Model file for the job. Use its own axes, mm. Coordinates: 2 decimals unless noted, no trailing zeros. Order: outer loops, then holes, each group sorted by start corner. A loop starts at its lowest first (then second) coordinate and runs counter-clockwise, first axis right, second up. Notation, with made-up numbers: (-19.5, 70) -> (36.5, 70) arc R8 cw to (36.5, 81) -> close; hole circle Ø5 at (-1.75, 18). An arc over 180 degrees is marked (long way). Use CSV: the item, a comma, the result in double quotes. Start each with the question number.
(1) Probe L1, parallel to Y at x = 40.9, z = -0.35; L2, parallel to X at y = 25.5, z = -0.75; L3, parallel to Z at x = -53, y = 20. List the from-to ranges inside material, lowest first.
(2) Cut at B-B on x = -21. Write the cut outline in (y, z), plus the area to 3 significant figures.
(3) Pull direction Y, two halves, no side cores. Call faces 1 (the cylindrical face through (-88.515, 24.98, -0.493)), 2 (the flat face through (-26.05, -0.584, -11.181)), 3 (the flat face through (-26, 18, -1)): pulls with the +Y half, pulls with the -Y half, needs draft (parallel to the pull), parting line crosses it, or undercut.
(4) Cut at C-C on y = -2.5. Write the cut outline in (x, z), plus the area to 3 significant figures.
(5) Pin check, flat tips, straight feed: pin 1 Ø4 at (x, y) = (-90.9, 24.23) entering from +Z; pin 2 Ø12 at (y, z) = (-2, -11) entering from -X; pin 3 Ø11 at (x, y) = (-32, 22.5) entering from -Z; pin 4 Ø6 at (x, y) = (-31.5, 8) entering from -Z. Stop position of each tip, or through.
(6) Cut at A-A on x = 40.9. Write the cut outline in (y, z).
```python
from build123d import *

# Parameters (mm, degrees)
SKETCH1_W            = 150
SKETCH1_H            = 23.35790613
BASE_FLANGE1_DEPTH   = 1
EDGE_FLANGE2_START   = -100
EDGE_FLANGE2_DEPTH   = 150
EDGE_FLANGE2_2_DEPTH = 150
SKETCH13_R           = 2.5
CUT_EXTRUDE1_DEPTH   = 3


# Read off the part's stored shape, not the designer's step: Edge-Flange2
# Sheet-metal steps are written as plain solids
with BuildPart() as part:
    # Sketch1 → Base-Flange1 (new body)
    with BuildSketch(Plane.XY):
        with Locations((-25, 17.550273337)):
            Rectangle(SKETCH1_W, SKETCH1_H)
    extrude(amount=-BASE_FLANGE1_DEPTH)

    # Edge-Flange2 outline → Edge-Flange2 (cut)
    with BuildSketch(Plane.YZ.offset(EDGE_FLANGE2_START)):
        with BuildLine():
            Line((5.871320272, 0), (5.871320272, -0.367006837))
            ThreePointArc((5.871320272, -0.367006837), (6.420209917, -0.093958772), (7.02602081, 0))
            Line((7.02602081, 0), (5.871320272, 0))
        make_face()
    extrude(amount=EDGE_FLANGE2_DEPTH, mode=Mode.SUBTRACT)

    # Edge-Flange2 2 outline → Edge-Flange2 2 (add)
    with BuildSketch(Plane.YZ.offset(EDGE_FLANGE2_START)):
        with BuildLine():
            ThreePointArc((5.871320272, -0.367006837), (5.548352573, -0.652225322), (5.293970003, -1))
            Line((5.293970003, -1), (-6.628679728, -21.650635095))
            Line((-6.628679728, -21.650635095), (-5.762654324, -22.150635095))
            Line((-5.762654324, -22.150635095), (6.159995406, -1.5))
            ThreePointArc((6.159995406, -1.5), (6.52602081, -1.133974596), (7.02602081, -1))
            Line((7.02602081, -1), (5.871320272, -1))
            Line((5.871320272, -1), (5.871320272, -0.367006837))
        make_face()
    extrude(amount=EDGE_FLANGE2_2_DEPTH)

    # Sketch13 → Cut-Extrude1 (cut)
    with BuildSketch(Plane.XY):
        with Locations((40.9, 24.229226402)):
            Circle(SKETCH13_R)
        with Locations((-90.9, 24.229226402)):
            Circle(SKETCH13_R)
    extrude(amount=-CUT_EXTRUDE1_DEPTH, mode=Mode.SUBTRACT)


solid = part.part
```
Outcome:
1,L1,"5.9 to 21.73, 26.73 to 29.23"
1,L2,"-100 to -93.05, -88.75 to 38.75, 43.05 to 50"
1,L3,"-1 to 0"
2,outline,"(-6.63, -21.65) -> (-5.76, -22.15) -> (6.16, -1.5) arc R1 cw to (7.03, -1) -> (29.23, -1) -> (29.23, 0) -> (7.03, 0) arc R2 ccw to (5.29, -1) -> close"
2,area,"47.6 mm2"
3,face 1,"undercut"
3,face 2,"pulls with the -Y half"
3,face 3,"needs draft"
4,outline,"(-100, -16.5) -> (50, -16.5) -> (50, -14.5) -> (-100, -14.5) -> close"
4,area,"300 mm2"
5,pin 1,"through"
5,pin 2,"x = -100"
5,pin 3,"z = -1"
5,pin 4,"z = -3.51"
6,outline,"(-6.63, -21.65) -> (-5.76, -22.15) -> (6.16, -1.5) arc R1 cw to (7.03, -1) -> (21.73, -1) -> (21.73, 0) -> (7.03, 0) arc R2 ccw to (5.29, -1) -> close; (26.73, -1) -> (29.23, -1) -> (29.23, 0) -> (26.73, 0) -> close"
